The listing builds one solid part. Answer for the finished solid, in the listing's coordinates (mm). A direction names the side the tool comes from. Coordinates: 2 decimals unless noted, no trailing zeros. Loops run counter-clockwise (first coordinate to the right, second up) from the corner with the lowest first, then second, coordinate; pieces in that order, holes last. Notation, with made-up numbers: (-1, 63) - (41, 63) arc R18 cw to (41, 91) - close; hole circle Ø2 at (-12.75, 51.5). An arc over 180 degrees is marked (long way). Return JSON: item names as keys, results as strings. Group by question number.
1. Find the intervals of material crossed by line 1 along Z through (x, y) = (0, 12.7); line 2 along X through (y, z) = (-4.25, -105); line 3 along Y through (x, z) = (-9.5, 104.5), in increasing order.
2. Section C-C (z = 152.5) is taken. Write down the section's boundary in (x, y).
3. Section B-B (x = -1) is taken. Write down the section's boundary in (y, z).
4. Section D-D (x = 22) is taken. Write down the section's boundary in (y, z).
5. This flat-tipped pin is pushed along its axis until it touches: P1, Ø2, axis at x = 18, z = -161, coming from the -Y side. Where does it stop, or does it pass through?
6. Section A-A (z = -218) is taken. Write down the section's boundary in (x, y), and give its area (4 significant figures).
7. Which of the six approach directions +Z, -Z, +X, -X, +Y, -Y give full straight-line access (tool end or side, diameter ignored) to faces 4 (the face through (-1.138, 13.479, -223.125)), 5 (the face through (0, 12, 4))?
8. The mould has two halves that part along X. Classify faces 1 (the face through (-30, 0, 4)), 2 (the face through (0, 15, 4)), 3 (the face through (-1.138, 13.479, -152.125)): pulls with the +X half, pulls with the -X half, needs draft (parallel to the pull), parting line crosses it, or undercut.
```python
from build123d import *

# Parameters (mm, degrees)
F1_DEPTH = 250
F3_D     = 10.5
F5_D     = 10.5


with BuildPart() as f1:
    # F0 (on Top) → F1 (new body, symmetric)
    with BuildSketch(Plane.XY):
        Polygon((30, 15), (-30, 15), (-30, -15), (-27, -15), (-27, 12), (27, 12), (27, -15), (30, -15), align=None)
    extrude(amount=F1_DEPTH, both=True)

    # F3 (through all)
    with Locations(Plane(origin=(0, 15, 0), x_dir=(-1, 0, 0), z_dir=(0, 1, 0))):
        with Locations((0, -218), (0, -147)):
            Hole(F3_D / 2)

    # F5 (through all)
    with Locations(Plane(origin=(0, 15, 0), x_dir=(-1, 0, 0), z_dir=(0, 1, 0))):
        with Locations((0, 220), (0, 40)):
            Hole(F5_D / 2)


solid = f1.part
```
The answers:
{
 "1": {"line 1": "z = -250 to -223.25, -212.75 to -152.25, -141.75 to 34.75, 45.25 to 214.75, 225.25 to 250", "line 2": "x = -30 to -27, 27 to 30", "line 3": "y = 12 to 15"},
 "2": {"outline": "(-30, -15) - (-27, -15) - (-27, 12) - (27, 12) - (27, -15) - (30, -15) - (30, 15) - (-30, 15) - close"},
 "3": {"outline": "(12, -250) - (15, -250) - (15, -223.15) - (12, -223.15) - close; (12, -212.85) - (15, -212.85) - (15, -152.15) - (12, -152.15) - close; (12, -141.85) - (15, -141.85) - (15, 34.85) - (12, 34.85) - close; (12, 45.15) - (15, 45.15) - (15, 214.85) - (12, 214.85) - close; (12, 225.15) - (15, 225.15) - (15, 250) - (12, 250) - close"},
 "4": {"outline": "(12, -250) - (15, -250) - (15, 250) - (12, 250) - close"},
 "5": {"P1": "stops at y = 12"},
 "6": {"outline": "(-30, -15) - (-27, -15) - (-27, 12) - (-5.25, 12) - (-5.25, 15) - (-30, 15) - close; (5.25, 12) - (27, 12) - (27, -15) - (30, -15) - (30, 15) - (5.25, 15) - close", "area": "310.5 mm2"},
 "7": {"face 4": "+Y, -Y", "face 5": "+Z, -Z, -Y"},
 "8": {"face 1": "pulls with the -X half", "face 2": "needs draft", "face 3": "undercut"}
}
